```python
from build123d import *

# Parameters (mm, degrees)
F0_W     = 6.35
F0_H     = 13.716
F1_DEPTH = 3.175
F0_W_2   = 1.5875
F0_H_2   = 73.952875
F2_DEPTH = 6.35
F0_W_3   = 46.9108536
F0_H_3   = 1.5875
F3_DEPTH = 11.684
F6_DEPTH = 3.81


# Not quite as in the source:
# - a feature names something its author has since deleted; it is built from what else it names


with BuildPart() as f1:
    # F0 (on Top) → F1 (new body)
    with BuildSketch(Plane.XY):
        Polygon((33.9837268, -49.6764375), (33.9837268, 49.6764375), (-33.9837268, 49.6764375), (-33.9837268, -24.2764375), (-12.9271268, -24.2764375), (-12.9271268, -49.6764375), align=None)
        with Locations((9.2978732, -40.2784375)):
            Rectangle(F0_W, F0_H, mode=Mode.SUBTRACT)
    extrude(amount=F1_DEPTH)

    # F0 (on Top) → F2 (join)
    with BuildSketch(Plane.XY):
        with Locations((-34.7774768, 12.7)):
            Rectangle(F0_W_2, F0_H_2)
    extrude(amount=F2_DEPTH)

    # F0 (on Top) → F3 (join)
    with BuildSketch(Plane.XY):
        with Locations((10.5283, -50.4701875)):
            Rectangle(F0_W_3, F0_H_3)
    extrude(amount=F3_DEPTH)

    # F5 (on face) → F6 (join)
    with BuildSketch(Plane.YZ.offset(33.9837268)):
        Polygon((-51.2639375, 13.3985), (-51.2639375, 11.684), (-49.6764375, 11.684), (49.6764375, 11.684), (49.6764375, 13.3985), align=None)
    extrude(amount=-F6_DEPTH)


solid = f1.part
```
Verification items for the finished model (mm, model axes). A direction names the side the tool comes from. Round coordinates to 2 decimals unless told otherwise and drop trailing zeros. Write each loop counter-clockwise with the first axis right and the second up, starting at its lowest first coordinate (ties: lowest second). Pieces come first, ordered by that corner, then holes. Notation, with made-up numbers: (59, -18.5) - (89, -18.5) arc R13 ccw to (89, -8.5) - close; hole circle Ø7 at (34.5, 42.25). An arc over 180 degrees is marked (long way). Answer as a JSON object with one key per item and string values. Group by question number.
Q1. Thickness scan on line 1 (Z direction, x = -30.5, y = -16.5) (3 decimals); line 2 (X direction, y = 31, z = 4); line 3 (Y direction, x = -5.5, z = 5.5). Record the ranges inside material, lowest first.
Q2. Section check D-D, the plane x = -24.5. Enter the section's corners in (y, z) (3 decimals).
Q3. Tool access check on faces 5 (the flat face through (-24, -24.276, 2)), 6 (the flat face through (9, -33.42, 2)), 7 (the flat face through (-35.571, 12, 3)), 8 (the flat face through (-33.984, 12, 5)), 9 (the flat face through (32, -1, 11.684)). Record the directions out of +Z, -Z, +X, -X, +Y, -Y that give a thin tool (end or side, any length) a straight path to the whole face; none if there is none.
Q4. Mould release check, pull along Y, two halves, no side actions. Record for faces 1 (the flat face through (-12.927, -41, 3)), 2 (the flat face through (-1, 49.676, 2)), 3 (the flat face through (9, -47.136, 2)), 4 (the flat face through (11, -51.264, 7)): released by +Y, released by -Y, zero draft, split by the parting line, or undercut.
Q5. Section check B-B, the plane z = 4.5. Enter the section's corners in (x, y).
Q6. Section check C-C, the plane y = -44.5. Enter the section's corners in (x, z) (1 decimal), plus the area to 3 significant figures.
Q7. Go/stop test with flat-tipped pins: pin 1 Ø7 at (x, z) = (-27, 4) entering from -Y; pin 2 Ø0.9 at (y, z) = (-26, 13) entering from -X; pin 3 Ø0.5 at (x, y) = (-35, 23.5) entering from +Z. Record where each tip stops, or that it passes through.
Found:
{
 "1": {"line 1": "z = 0 to 3.175", "line 2": "x = -35.57 to -33.98", "line 3": "y = -51.26 to -49.68"},
 "2": {"outline": "(-24.276, 0) - (49.676, 0) - (49.676, 3.175) - (-24.276, 3.175) - close"},
 "3": {"face 5": "+Z, -Z, -X, -Y", "face 6": "+Z, -Z", "face 7": "+Z, -Z, -X, +Y, -Y", "face 8": "+Z, +X, +Y, -Y", "face 9": "+X, -X, +Y"},
 "4": {"face 1": "zero draft", "face 2": "released by +Y", "face 3": "undercut", "face 4": "released by -Y"},
 "5": {"outline": "(-35.57, -24.28) - (-33.98, -24.28) - (-33.98, 49.68) - (-35.57, 49.68) - close; (-12.93, -51.26) - (33.98, -51.26) - (33.98, -49.68) - (-12.93, -49.68) - close"},
 "6": {"outline": "(-12.9, 0) - (6.1, 0) - (6.1, 3.2) - (-12.9, 3.2) - close; (12.5, 0) - (34, 0) - (34, 3.2) - (12.5, 3.2) - close; (30.2, 11.7) - (34, 11.7) - (34, 13.4) - (30.2, 13.4) - close", "area": "135 mm^2"},
 "7": {"pin 1": "stops at y = -24.28", "pin 2": "stops at x = 30.17", "pin 3": "stops at z = 6.35"}
}
